Source: three-view drawing plus pictorial views. Frame: mm from the lowest corner of the part. A direction names the side the tool comes from. Give positions to 0.01 mm unless a question says otherwise; leave off trailing zeros. Loops run counter-clockwise (first coordinate to the right, second up) from the corner with the lowest first, then second, coordinate; pieces in that order, holes last. Notation, with made-up numbers: M 17.25,79.5 L 23.25,79.5 A28 cw 23.25,98.5 Z; hole C 46,12 d10. An arc over 180 degrees is marked long. Write item = value, one per line.
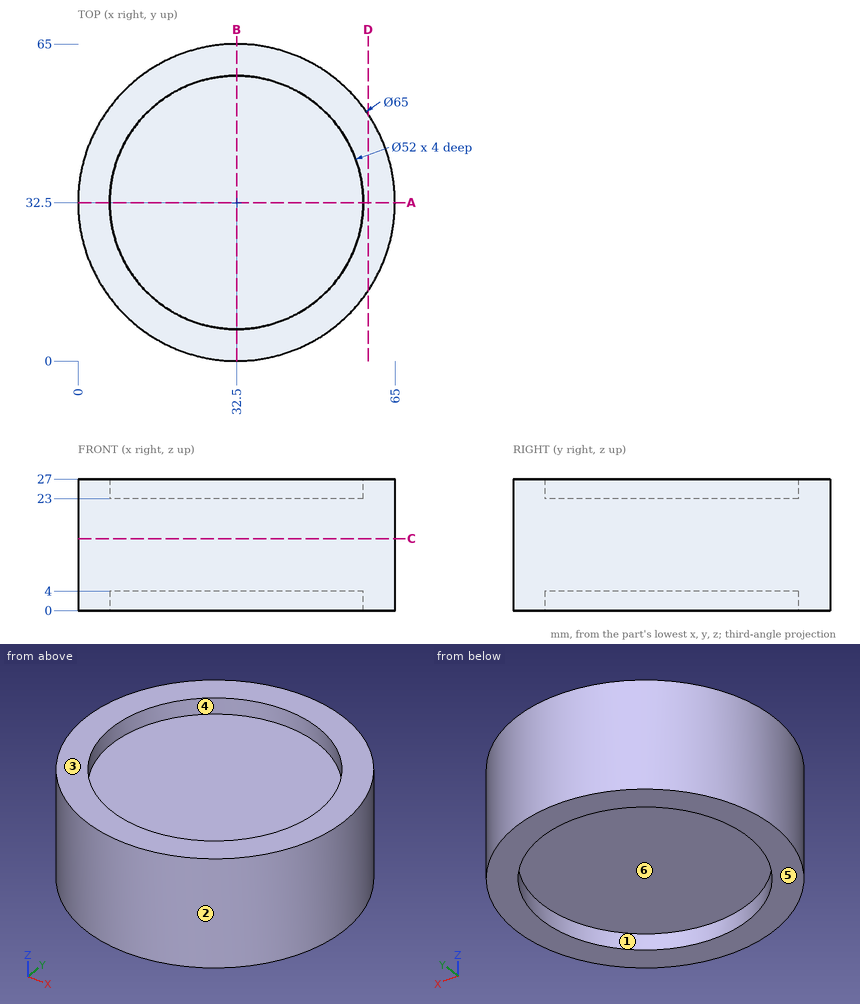
1. Cut plane C-C, the plane z = 14.75. Return the cut outline in (x, y).
Derived:
outline = C 32.5,32.5 d65
2. First-contact query: pin 1 Ø4 at (y, z) = (19.5, 9.5) entering from -X; pin 2 Ø6 at (x, z) = (30.5, 9.5) entering from +Y; pin 3 Ø2 at (x, z) = (56, 7.5) entering from +Y. Flat tips, straight axial feed; report the tip coordinate or a pass-through.
Derived:
pin_1 = 1.92
pin_2 = 65
pin_3 = 55.95
3. Reachability of the marked faces 4, 5 and 6 from +Z, -Z, +X, -X, +Y, -Y: full face, straight path, thin tool, end or side. Return the list, or none.
Derived:
face_4 = +Z
face_5 = -Z, +X, -X, +Y, -Y
face_6 = -Z
4. Cut plane D-D, the plane x = 59.5. Return the cut outline in (y, z).
Derived:
outline = M 14.41,0 L 50.59,0 L 50.59,27 L 14.41,27 Z
5. Cut plane A-A, the plane y = 32.5. Return the cut outline in (x, z).
Derived:
outline = M 0,0 L 6.5,0 L 6.5,4 L 58.5,4 L 58.5,0 L 65,0 L 65,27 L 58.5,27 L 58.5,23 L 6.5,23 L 6.5,27 L 0,27 Z
6. Material intervals for probe 1 along Y at (x, z) = (32.5, 2.2); probe 2 along Z at (x, y) = (43, 39); probe 3 along X at (y, z) = (53, 23.25), sorted ascending. Write a range as from..to.
Derived:
probe_1 = 0..6.5, 58.5..65
probe_2 = 4..23
probe_3 = 7.28..16.51, 48.49..57.72
7. Pull-direction query (Y, two-part tool) for the marked faces 1, 2 and 3; classes: +Y half, -Y half, draft (parallel to the pull), parting line (faces both ways), or undercut.
Derived:
face_1 = undercut
face_2 = parting line
face_3 = draft
